Here's how the part is built. I have some questions about the finished solid (model axes, mm). A direction names the side the tool comes from. Round coordinates to 2 decimals unless told otherwise and drop trailing zeros. Write each loop counter-clockwise with the first axis right and the second up, starting at its lowest first coordinate (ties: lowest second). Pieces come first, ordered by that corner, then holes. Notation, with made-up numbers: (71.25, 52) - (106.25, 52) arc R23 cw to (106.25, 61) - close; hole circle Ø2 at (82.5, 72.5). An arc over 180 degrees is marked (long way). One line per item, written item: value. Start each with the question number.
Item 1: Imagine slicing it at D-D, the plane y = 11.25. Please give me the cut outline in (x, z) (3 decimals), then the cut area to 3 significant figures.
Item 2: Imagine slicing it at B-B, the plane z = 3.75. Please give me the cut outline in (x, y), then the cut area to 3 significant figures.
Item 3: Imagine slicing it at C-C, the plane x = -1.5. Please give me the cut outline in (y, z).
Item 4: Imagine slicing it at A-A, the plane y = -0.75. Please give me the cut outline in (x, z) (3 decimals).
Item 5: Thinking about a two-plate mould opening in Y: for faces 1 (the face through (10, 12.7, 17)), 2 (the face through (4, 0, 0)), 3 (the face through (12.656, -0.112, 17.663)), which applies, released by +Y, released by -Y, zero draft, split by the parting line, or undercut?
Item 6: For faces 4 (the face through (-4.213, 0.176, 11.116)), 5 (the face through (11, 0, 10.16)), 6 (the face through (9.525, 0, 24)), which set-ups out of +Z, -Z, +X, -X, +Y, -Y let a thin tool reach every point of the face, with its end or its side?
Item 7: If I drill on line 1 (Z direction, x = -3.75, y = 0); line 2 (X direction, y = -5.75, z = 23.25) (3 decimals); line 3 (Y direction, x = 0, z = 6.25), over which ranges is the centre line in solid material (lowest first)?
Item 8: For P1, Ø12, axis at x = -0.5, y = -6.5, coming from the +Z side; P2, Ø2, axis at x = -9.5, y = -1.5, coming from the +Z side; P3, Ø8, axis at x = -2.5, z = 6, coming from the -Y side, each with a flat end and sliding along its axis, tell me the tip position at first contact or that it passes through.
Autodesk Inventor part; units mm, degrees
ref_plane "YZ Plane" through (0, 0, 0) normal (1, 0, 0) x (0, 1, 0)
ref_plane "XZ Plane" through (0, 0, 0) normal (0, 1, 0) x (-1, 0, 0)
ref_plane "XY Plane" through (0, 0, 0) normal (0, 0, 1) x (1, 0, 0)
sketch "Sketch1" plane through (0, 0, 0) normal (0, 0, 1) x (1, 0, 0)
  circle A0 centre (0, 0) radius 10.16
  circle A1 centre (0, 0) radius 8.7376
  dimension "d0" = 20.32
  dimension "d6" = 17.4752
extrude "Extrusion1" add sketch "Sketch1" along normal blind 10.16 contours A0 | A1
sketch "Sketch2" plane through (0, 0, 10.16) normal (0, 0, 1) x (1, 0, 0)
  circle A0 centre (0, 0) radius 10.16
  circle A1 centre (0, 0) radius 12.7 construction
  line L0 (0, 12.7) -> (15.875, 12.7)
  line L1 (15.875, 12.7) -> (15.875, -12.7)
  line L2 (15.875, -12.7) -> (0, -12.7)
  arc A2 (0, 12.7) -> (0, -12.7) centre (0, 0) ccw
  point P0 (15.875, 0)
  dimension "d3" = 2.54
  dimension "d14" = 15.875
  dimension "d35" = 25.4
extrude "Extrusion2" add sketch "Sketch2" along normal blind 6.35 contours A0 | L0 L1 L2 A2
sketch "Sketch4" plane through (0, 0, 16.51) normal (0, 0, 1) x (1, 0, 0)
  arc A0 (0, 12.7) -> (0, -12.7) centre (0, 0) ccw
hole "Hole2" at (0, 0, 16.51) direction (0, 0, -1) diameter 6.5278 end through all
sketch "Sketch5" plane through (0, 0, 16.51) normal (0, 0, 1) x (1, 0, 0)
  line L0 (15.875, 12.7) -> (0, 12.7)
  line L1 (0, -12.7) -> (15.875, -12.7)
  line L2 (15.875, 12.7) -> (9.525, 12.7)
  line L3 (9.525, 12.7) -> (9.525, -12.7)
  line L4 (9.525, -12.7) -> (15.875, -12.7)
  line L5 (15.875, -12.7) -> (15.875, 12.7)
  point P0 (0, 0)
  dimension "d22" = 6.35
extrude "Extrusion3" add sketch "Sketch5" along normal blind 12.7
fillet "Fillet1" radius 3.175 1 edges at (9.525, 0, 16.51)
sketch "Sketch6" plane through (15.875, -12.7, 10.16) normal (1, 0, 0) x (0, 0, -1)
  line L0 (-12.7, 19.05) -> (-12.7, 6.35) construction
  line L1 (-19.05, 0) -> (-19.05, 25.4) construction
  line L2 (0, 25.4) -> (-19.05, 25.4) construction
  point P0 (10.16, 12.7)
  point P1 (-12.7, 12.7)
  point P2 (-19.05, 12.7)
  point P3 (-9.525, 25.4)
  point P4 (-4.953, 12.7)
  dimension "d26" = 12.7
  dimension "d34" = 6.35
  dimension "d36" = 14.097
hole "Hole3" at (15.875, 0, 15.113) direction (-1, 0, 0) diameter 5.1054 end through all
ref_plane "Work Plane1" through (-12.7, -12.7, 29.21) normal (-1, 0, 0) x (0, 0, 1)
sketch "Sketch7" plane through (-12.7, -12.7, 29.21) normal (-1, 0, 0) x (0, 0, 1)
  line L0 (-19.05, 12.7) -> (-16.6497, 12.7) construction
  line L1 (-19.05, 12.7) -> (-16.6497, 12.7) construction
  circle A0 centre (-14.097, 12.7) radius 2.5527 construction
  circle A1 centre (-14.097, 12.7) radius 4.0005
  point P0 (-29.21, 12.7)
  point P1 (-12.7, 10.5635)
  point P2 (-12.7, 14.8365)
  dimension "d38" = 8.001
extrude "Extrusion4" cut sketch "Sketch7" against normal up to surface (22.225 mm away)
properties part number "constant force Spring Holder 2" material "ABS Plastic"
Values follow:
1. outline: (-5.893, 10.16) - (15.875, 10.16) - (15.875, 29.21) - (9.525, 29.21) - (9.525, 19.685) arc R3.175 cw to (6.35, 16.51) - (-5.893, 16.51) - close
1. area: 221 mm^2
2. outline: circle Ø20.32 at (0, 0); hole circle Ø6.53 at (0, 0)
2. area: 291 mm^2
3. outline: (-12.61, 10.16) - (-10.05, 10.16) - (-10.05, 0) - (-2.9, 0) - (-2.9, 12.36) arc R4 cw to (-3.75, 16.51) - (-12.61, 16.51) - close; (2.9, 0) - (10.05, 0) - (10.05, 10.16) - (12.61, 10.16) - (12.61, 16.51) - (3.75, 16.51) arc R4 cw to (2.9, 12.36) - close
4. outline: (-12.678, 10.16) - (-10.132, 10.16) - (-10.132, 0) - (-3.177, 0) - (-3.177, 11.183) - (-12.678, 11.183) - close; (3.177, 0) - (10.132, 0) - (10.132, 10.16) - (15.875, 10.16) - (15.875, 12.673) - (9.525, 12.673) - (9.525, 11.183) - (3.177, 11.183) - close; (9.459, 19.043) - (9.525, 19.043) - (9.525, 17.553) - (15.875, 17.553) - (15.875, 29.21) - (9.525, 29.21) - (9.525, 19.685) arc R3.175 cw to start
5. face 1: released by +Y
5. face 2: zero draft
5. face 3: undercut
6. face 4: -X
6. face 5: -Z
6. face 6: +Z, -X, +Y, -Y
7. line 1: z = 0 to 11.11
7. line 2: x = 9.525 to 15.875
7. line 3: y = -10.16 to -3.26, 3.26 to 10.16
8. P1: stops at z = 16.51
8. P2: stops at z = 11.99
8. P3: stops at y = -10.16
